Source: CAD feature listing. Evaluate the final solid. Frame: model axes, mm. A direction names the side the tool comes from. Coordinates: 2 decimals unless noted, no trailing zeros. Write each loop counter-clockwise with the first axis right and the second up, starting at its lowest first coordinate (ties: lowest second). Pieces come first, ordered by that corner, then holes. Notation, with made-up numbers: (-0.5, 89.25) -> (4.5, 89.25) arc R30 ccw to (4.5, 126.25) -> close; hole circle Ø5 at (-17, 20). An arc over 180 degrees is marked (long way). One line per item, written item: value. Start each with the question number.
1. Mould query, pull axis Z, two halves, no side actions, for faces 1 (the flat face through (-11, 11, -22)), 2 (the cylindrical face through (6.94, 7.4, 31.24)), 3 (the flat face through (7.7, -46, -15.5)). Classes: released by +Z, released by -Z, zero draft, split by the parting line, or undercut.
2. First-contact query: P1, Ø12, axis at x = 10.5, y = -8.5, coming from the +Z side; P2, Ø1.5, axis at y = -0.5, z = 25.5, coming from the +X side; P3, Ø5, axis at y = -14.5, z = 19.5, coming from the -X side. Flat tips, straight axial feed; report the tip coordinate or a pass-through.
3. Access query for faces 4 (the cylindrical face through (23.846, -20.706, -7.509)), 5 (the flat face through (10.3, 7, 10.3)), 6 (the cylindrical face through (-4.336, -22.028, -19.524)). Directions: +Z, -Z, +X, -X, +Y, -Y. A direction counts if a zero-diameter tool reaches every point of the face in a straight line with its end or side. Return the directions, or none.
4. Line query: line 1 (Y direction, x = 8.5, z = 16); line 2 (Z direction, x = 0, y = -7.25); line 3 (Z direction, x = 0, y = 13.15). Output: solid intervals per line, ascending.
5. Section query C-C, the plane y = -25. Output: boundary loops of the cut face in (x, z).
6. Section query D-D, the plane z = -27. Output: boundary loops of the cut face in (x, y).
Autodesk Inventor part; units mm, degrees
ref_plane "YZ Plane" through (0, 0, 0) normal (1, 0, 0) x (0, 1, 0)
ref_plane "XZ Plane" through (0, 0, 0) normal (0, 1, 0) x (-1, 0, 0)
ref_plane "XY Plane" through (0, 0, 0) normal (0, 0, 1) x (1, 0, 0)
sketch "Sketch1" plane through (0, 0, 0) normal (0, 1, 0) x (-1, 0, 0)
  circle A0 centre (0, 0) radius 32
  dimension "d0" = 64
extrude "Extrusion1" add sketch "Sketch1" along normal blind 15
sketch "Sketch2" plane through (0, 15, 0) normal (0, 1, 0) x (1, 0, 0)
  point P0 (0, 0)
sketch "Sketch3" plane through (0, 0, 0) normal (0, -1, 0) x (1, 0, 0)
  circle A0 centre (0, 0) radius 25
  dimension "d3" = 50
extrude "Extrusion2" add sketch "Sketch3" along normal blind 46
sketch "Sketch4" plane through (0, 15, 0) normal (0, 1, 0) x (1, 0, 0)
  circle A0 centre (0, 0) radius 29
  dimension "d6" = 58
extrude "Extrusion3" cut sketch "Sketch4" against normal blind 4
sketch "Sketch5" plane through (0, 11, 0) normal (0, 1, 0) x (1, 0, 0)
  circle A0 centre (0, 0) radius 24
  dimension "d9" = 48
extrude "Extrusion4" cut sketch "Sketch5" against normal blind 4
sketch "Sketch6" plane through (0, 7, 0) normal (0, 1, 0) x (1, 0, 0)
  point P0 (0, 0)
sketch "Sketch7" plane through (0, -46, 0) normal (0, -1, 0) x (1, 0, 0)
  circle A0 centre (0, 0) radius 17
  dimension "d12" = 34
extrude "Extrusion5" cut sketch "Sketch7" against normal blind 22
sketch "Sketch8" plane through (0, -24, 0) normal (0, -1, 0) x (1, 0, 0)
  circle A0 centre (0, 0) radius 20
  dimension "d15" = 40
extrude "Extrusion6" cut sketch "Sketch8" against normal blind 4
sketch "Sketch9" plane through (0, 7, 0) normal (0, 1, 0) x (1, 0, 0)
  circle A0 centre (0, 0) radius 14
  dimension "d18" = 28
extrude "Extrusion7" cut sketch "Sketch9" against normal blind 27
chamfer "Chamfer1" distance 4 angle 45 1 edges at (-25, -46, 0)
properties part number "00.32.002 \"Fitting\"" material "Steel"
Computed values:
1. face 1: undercut
1. face 2: split by the parting line
1. face 3: zero draft
2. P1: stops at z = 24.59
2. P2: stops at x = 20.05
2. P3: stops at x = -18.33
3. face 4: -Y
3. face 5: +Y
3. face 6: none
4. line 1: y = -46 to -24, -20 to 7
4. line 2: z = -25 to -14, 14 to 25
4. line 3: z = -32 to -29, 29 to 32
5. outline: circle Ø50 at (0, 0); hole circle Ø34 at (0, 0)
6. outline: (-17.18, 0) -> (17.18, 0) -> (17.18, 15) -> (10.58, 15) -> (10.58, 11) -> (-10.58, 11) -> (-10.58, 15) -> (-17.18, 15) -> close
